```python
from build123d import *

# Parameters (mm, degrees)
SKETCH_1_W          = 2200
SKETCH_1_H          = 60
EXTRUDE_1_DEPTH     = 5
CHAMFER_1_SIZE      = 5
CHAMFER_1_SIZE_2    = 10
SKETCH_2_W          = 2200
SKETCH_2_H          = 5
CUT_EXTRUDE_2_DEPTH = 3


with BuildPart() as part:
    # Эскиз1 → Бобышка-Вытянуть1 (new body)
    with BuildSketch(Plane.XY):
        with Locations((1100, -30)):
            Rectangle(SKETCH_1_W, SKETCH_1_H)
    extrude(amount=EXTRUDE_1_DEPTH)

    # Фаска1
    # the kernel refuses this chamfer: 10, 5 mm, written as the material it takes off along each edge
    with BuildSketch(Plane(origin=(2225.898288738, 0, 5), x_dir=(0, 0.06891834360170877, -0.9976223042390326), z_dir=(-1, 0, 0)), Plane(origin=(-25.898288738, -60, 5), x_dir=(0, -0.06891834360170909, -0.9976223042390324), z_dir=(1, 0, 0))) as chamfer_1_piece_1:
        Polygon((CHAMFER_1_SIZE * 0.997622304239, CHAMFER_1_SIZE * 0.0689183436017), (-CHAMFER_1_SIZE_2 * 0.0689183436017, CHAMFER_1_SIZE_2 * 0.997622304239), (0, 0), align=None)
    extrude(amount=2251.796577476, mode=Mode.SUBTRACT)

    # Эскиз2 → Вырез-Вытянуть2 (cut)
    with BuildSketch(Plane.XY.offset(5)):
        with Locations((1100, -46.5)):
            Rectangle(SKETCH_2_W, SKETCH_2_H)
        with Locations((1100, -13.5)):
            Rectangle(SKETCH_2_W, SKETCH_2_H)
    extrude(amount=-CUT_EXTRUDE_2_DEPTH, mode=Mode.SUBTRACT)


solid = part.part
```
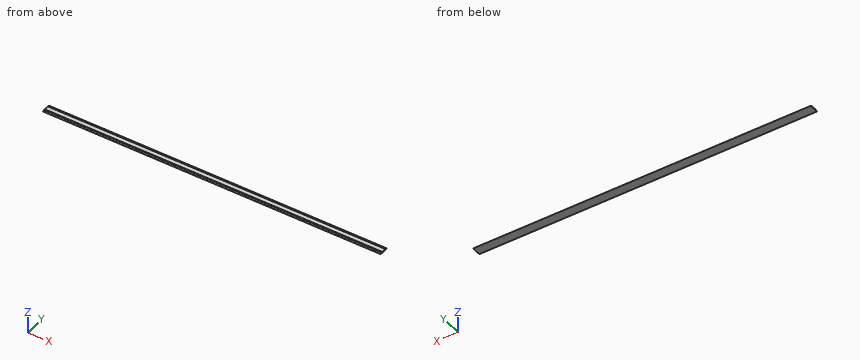
Source: CAD feature listing. Evaluate the final solid. Frame: model axes, mm. Round coordinates to 2 decimals unless told otherwise and drop trailing zeros. Loops run counter-clockwise (first coordinate to the right, second up) from the corner with the lowest first, then second, coordinate; pieces in that order, holes last.
1. Contact query for flat-ended pins moving along their axis: pin 1 (2.5 mm diameter, centred on x = 781, z = 3.5, fed in from +Y); pin 2 (0.9 mm diameter, centred on x = 1206, z = 4, fed in from -Y); pin 3 (0.9 mm diameter, centred on x = 1038.5, z = 3.5, fed in from +Y). Output: stop coordinate, or through.
2. Section query B-B on x = 2032. Output: boundary loops of the cut face in (y, z).
3. Section query A-A on z = 3.3. Output: boundary loops of the cut face in (x, y), and give its area (3 significant figures).
4. Ray query, L1, parallel to Y at x = 174, z = 2.2; L2, parallel to Y at x = 986, z = 3.25; L3, parallel to Z at x = 1382, y = -3.5. Return the intervals inside material, ascending.
Answers below:
1. pin 1: stops at y = -4.5
1. pin 2: stops at y = -52.9
1. pin 3: stops at y = -6.1
2. outline: (-60, 0) - (0, 0) - (-10, 5) - (-11, 5) - (-11, 2) - (-16, 2) - (-16, 5) - (-44, 5) - (-44, 2) - (-49, 2) - (-49, 5) - (-50, 5) - close
3. outline: (0, -53.4) - (2200, -53.4) - (2200, -49) - (0, -49) - close; (0, -44) - (2200, -44) - (2200, -16) - (0, -16) - close; (0, -11) - (2200, -11) - (2200, -6.6) - (0, -6.6) - close
3. area: 81,000 mm2
4. L1: y = -55.6 to -49, -44 to -16, -11 to -4.4
4. L2: y = -53.5 to -49, -44 to -16, -11 to -6.5
4. L3: z = 0 to 1.75
